from build123d import *

# Parameters (mm, degrees)
SKETCH_1_R          = 55
EXTRUDE_1_DEPTH     = 5
SKETCH_5_W          = 47
SKETCH_5_H          = 12.24289715
CUT_EXTRUDE_2_DEPTH = 30
FILLET_4_R          = 2
FILLET_5_R          = 2
EXTRUDE_START       = -3
EXTRUDE_3_DEPTH     = 3
FILLET_7_R          = 10
FILLET_8_R          = 5
SKETCH_10_R         = 3
CUT_EXTRUDE_5_DEPTH = 3
SKETCH_15_R         = 6.7
CUT_EXTRUDE_6_DEPTH = 10
SKETCH_16_R         = 2
CUT_EXTRUDE_7_DEPTH = 10


with BuildPart() as part:
    # 草图1 → 凸台-拉伸1 (new body)
    with BuildSketch(Plane(origin=(0, 0, 0), x_dir=(1, 0, 0), z_dir=(0, 1, 0))):
        with Locations(Location((0, 0, 0), (0, 0, 270))):
            Circle(SKETCH_1_R)
    extrude(amount=EXTRUDE_1_DEPTH)

    # 草图5 → 切除-拉伸2 (cut)
    with BuildSketch(Plane(origin=(0, 5, 0), x_dir=(1, 0, 0), z_dir=(0, 1, 0))):
        with Locations((0, 49.687490397)):
            Rectangle(SKETCH_5_W, SKETCH_5_H)
    extrude(amount=-CUT_EXTRUDE_2_DEPTH, mode=Mode.SUBTRACT)

    # 圆角4
    fillet_4_edges = [part.edges().sort_by_distance(p)[0] for p in [
        (-23.5, 2.5, -49.726753363),
    ]]
    fillet(fillet_4_edges, radius=FILLET_4_R)

    # 圆角5
    fillet_5_edges = [part.edges().sort_by_distance(p)[0] for p in [
        (23.5, 2.5, -49.726753363),
    ]]
    fillet(fillet_5_edges, radius=FILLET_5_R)

    # 草图14 → 凸台-拉伸3 (add)
    with BuildSketch(Plane(origin=(0, 3, 0), x_dir=(1, 0, 0), z_dir=(0, 1, 0)).offset(EXTRUDE_START)):
        with BuildLine():
            Line((-49.898576095, 23.132922507), (-63.862525635, 37.044772973))
            Line((-63.862525635, 37.044772973), (-49.746845912, 51.213315099))
            Line((-49.746845912, 51.213315099), (-38.128637352, 39.638453724))
            ThreePointArc((-38.128637352, 39.638453724), (-44.78063998, 31.932652301), (-49.898576095, 23.132922507))
        make_face()
        with BuildLine():
            Line((49.811900188, -23.3189751), (64.421720913, -37.928795825))
            Line((64.421720913, -37.928795825), (50.279585289, -52.070931449))
            Line((50.279585289, -52.070931449), (37.984884655, -39.776230814))
            ThreePointArc((37.984884655, -39.776230814), (44.662950793, -32.097053236), (49.811900188, -23.3189751))
        make_face()
        with BuildLine():
            Line((-49.632393674, -23.698639164), (-63.862550335, -37.928795825))
            Line((-63.862550335, -37.928795825), (-49.720414711, -52.070931449))
            Line((-49.720414711, -52.070931449), (-37.697852746, -40.048369484))
            ThreePointArc((-37.697852746, -40.048369484), (-44.423770724, -32.427281642), (-49.632393674, -23.698639164))
        make_face()
        with BuildLine():
            Line((38.475737251, 39.301623923), (50.118901666, 51.212426922))
            Line((50.118901666, 51.212426922), (64.420808036, 37.231887798))
            Line((64.420808036, 37.231887798), (50.134465219, 22.6171483))
            ThreePointArc((50.134465219, 22.6171483), (45.083643676, 31.50341367), (38.475737251, 39.301623923))
        make_face()
    extrude(amount=EXTRUDE_3_DEPTH)

    # 圆角7
    fillet_7_edges = [part.edges().sort_by_distance(p)[0] for p in [
        (-38.128637352, 1.5, -39.638453724),
        (-49.898576095, 1.5, -23.132922507),
        (-49.632393674, 1.5, 23.698639164),
        (-37.697852746, 1.5, 40.048369484),
        (50.134465219, 1.5, -22.6171483),
        (38.475737251, 1.5, -39.301623923),
        (37.984884655, 1.5, 39.776230814),
        (49.811900188, 1.5, 23.3189751),
    ]]
    fillet(fillet_7_edges, radius=FILLET_7_R)

    # 圆角8
    fillet_8_edges = [part.edges().sort_by_distance(p)[0] for p in [
        (-63.862525635, 1.5, -37.044772973),
        (-49.746845912, 1.5, -51.213315099),
        (-49.720414711, 1.5, 52.070931449),
        (-63.862550335, 1.5, 37.928795825),
        (50.118901666, 1.5, -51.212426922),
        (64.420808036, 1.5, -37.231887798),
        (50.279585289, 1.5, 52.070931449),
        (64.421720913, 1.5, 37.928795825),
    ]]
    fillet(fillet_8_edges, radius=FILLET_8_R)

    # 草图10 → 切除-拉伸5 (cut)
    with BuildSketch(Plane(origin=(0, 3, 0), x_dir=(1, 0, 0), z_dir=(0, 1, 0))):
        with Locations(Location((-49.720414711, 37.071204175, 0), (0, 0, 270))):
            Circle(SKETCH_10_R)
        with Locations(Location((50.279585289, 37.071204175, 0), (0, 0, 270))):
            Circle(SKETCH_10_R)
        with Locations(Location((-49.720414711, -37.928795825, 0), (0, 0, 270))):
            Circle(SKETCH_10_R)
        with Locations(Location((50.279585289, -37.928795825, 0), (0, 0, 270))):
            Circle(SKETCH_10_R)
    extrude(amount=-CUT_EXTRUDE_5_DEPTH, mode=Mode.SUBTRACT)

    # 草图15 → 切除-拉伸6 (cut)
    with BuildSketch(Plane(origin=(0, 5, 0), x_dir=(1, 0, 0), z_dir=(0, 1, 0))):
        with Locations(Location((0, 0, 0), (0, 0, 270))):
            Circle(SKETCH_15_R)
    extrude(amount=-CUT_EXTRUDE_6_DEPTH, mode=Mode.SUBTRACT)

    # 草图16 → 切除-拉伸7 (cut)
    with BuildSketch(Plane(origin=(0, 5, 0), x_dir=(1, 0, 0), z_dir=(0, 1, 0))):
        with Locations(Location((-26, 0, 0), (0, 0, 270))):
            Circle(SKETCH_16_R)
        with Locations(Location((26, 0, 0), (0, 0, 270))):
            Circle(SKETCH_16_R)
    extrude(amount=-CUT_EXTRUDE_7_DEPTH, mode=Mode.SUBTRACT)


solid = part.part
Geometry: final body of the model. Coordinates: model frame, mm. A direction names the side the tool comes from. Coordinates: 2 decimals unless noted, no trailing zeros. Order: outer loops, then holes, each group sorted by start corner. A loop starts at its lowest first (then second) coordinate and runs counter-clockwise, first axis right, second up.
(1) First-contact query: pin 1 (8 mm diameter, centred on x = 50.28, z = -37.07, fed in from +Y); pin 2 (5 mm diameter, centred on x = -26, z = 0, fed in from -Y); pin 3 (1.5 mm diameter, centred on y = 3.5, z = -22.5, fed in from +X); pin 4 (1.5 mm diameter, centred on x = 6, y = 0.5, fed in from -Z). Flat tips, straight axial feed; report the tip coordinate or a pass-through.
(2) Section query D-D (z = -12.5). Return the cut outline in (x, y).
(3) Draft query along X for faces 1 (the face through (52.019, 1.521, -22.414)), 2 (the face through (1, 5, -9)), 3 (the face through (24, 3, 0)). Return one class per face: pulls with the +X half, pulls with the -X half, needs draft (parallel to the pull), parting line crosses it, or undercut.
(4) Section query B-B (z = 0). Return the cut outline in (x, y), plus the area to 3 significant figures.
(5) Section query C-C (y = 0.9). State how many separate pieces and enclosed holes the cut face has, plus the area to 3 significant figures.
(6) Access query for faces 4 (the face through (-57.4, 1.479, -30.606)), 5 (the face through (57.635, 1.479, 31.142)), 6 (the face through (47, 3, 37)). Directions: +Z, -Z, +X, -X, +Y, -Y. A direction counts if a zero-diameter tool reaches every point of the face in a straight line with its end or side. Return the directions, or none.
(7) Section query A-A (x = 0). Return the cut outline in (y, z), plus the area to 3 significant figures.
(8) Material intervals for probe 1 along X at (y, z) = (1.9, 38); probe 2 along X at (y, z) = (3.1, 0); probe 3 along X at (y, z) = (2.1, 44.5), sorted ascending.
Solution:
1. pin 1: stops at y = 3
1. pin 2: stops at y = 0
1. pin 3: stops at x = 52.19
1. pin 4: stops at z = -43.57
2. outline: (-53.56, 0) - (53.56, 0) - (53.56, 5) - (-53.56, 5) - close
3. face 1: pulls with the +X half
3. face 2: needs draft
3. face 3: undercut
4. outline: (-55, 0) - (-28, 0) - (-28, 5) - (-55, 5) - close; (-24, 0) - (-6.7, 0) - (-6.7, 5) - (-24, 5) - close; (6.7, 0) - (24, 0) - (24, 5) - (6.7, 5) - close; (28, 0) - (55, 0) - (55, 5) - (28, 5) - close
4. area: 443 mm2
5. separate pieces: 1
5. enclosed holes: 7
5. area: 10,200 mm2
6. face 4: -X, +Y, -Y
6. face 5: +X, +Y, -Y
6. face 6: +Z, +X, +Y
7. outline: (0, -43.57) - (5, -43.57) - (5, -6.7) - (0, -6.7) - close; (0, 6.7) - (5, 6.7) - (5, 55) - (0, 55) - close
7. area: 426 mm2
8. probe 1: x = -61.79 to -52.72, -46.72 to 47.28, 53.28 to 62.35
8. probe 2: x = -55 to -28, -24 to -6.7, 6.7 to 24, 28 to 55
8. probe 3: x = -57.29 to -41.41, -32.53 to 32.43, 42.17 to 57.85
